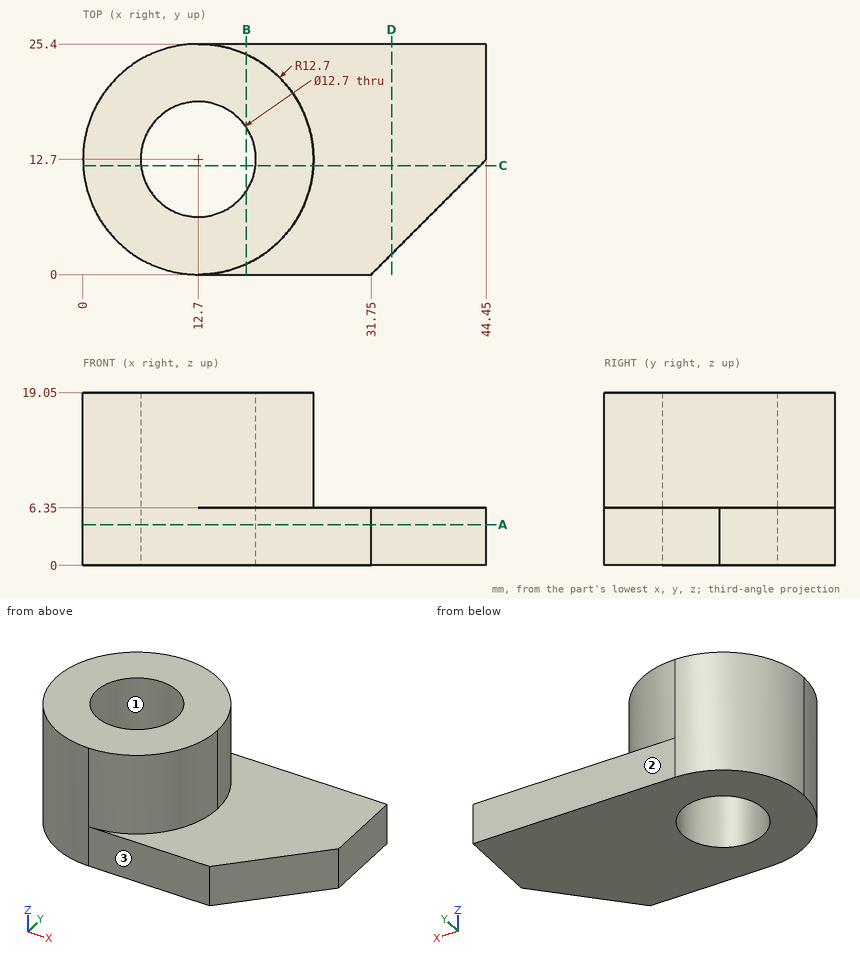
Geometry: see drawing. Coordinates: mm, zero at the bounding-box minimum. Coordinates: 2 decimals unless noted, no trailing zeros. Order: outer loops, then holes, each group sorted by start corner. A loop starts at its lowest first (then second) coordinate and runs counter-clockwise, first axis right, second up. Notation, with made-up numbers: M 85.25,17 L 89.25,17 A15 ccw 89.25,40 Z; hole C 88,81.5 d9. An arc over 180 degrees is marked long. Write each question's results on one line, items separated by ' | '. Start each with the question number.
1) Section query A-A (z = 4.5). Return the cut outline in (x, y).
2) Line query: line 1 (Z direction, x = 25, y = 7.25); line 2 (X direction, y = 13.5, z = 7); line 3 (Y direction, x = 18, z = 5.25). Output: solid intervals per line, ascending. Write a range as from..to.
3) Section query B-B (x = 18). Return the cut outline in (y, z).
4) Section query D-D (x = 34). Return the cut outline in (y, z), plus the area to 3 significant figures.
5) Draft query along Y for the marked faces 1, 2 and 3. Return one class per face: released by +Y, released by -Y, zero draft, split by the parting line, or undercut.
6) Contact query for flat-ended pins moving along their axis: pin 1 Ø3 at (y, z) = (16.5, 3.5) entering from -X; pin 2 Ø4 at (y, z) = (13.5, 13) entering from +X; pin 3 Ø1 at (x, z) = (23, 8) entering from +Y; pin 4 Ø1 at (x, y) = (17, 16.5) entering from +Z. Output: stop coordinate, or through.
7) Section query C-C (y = 12). Return the cut outline in (x, z).
Answers:
1) outline: M 12.7,0 L 31.75,0 L 44.45,12.7 L 44.45,25.4 L 12.7,25.4 A12.7 ccw Z; hole C 12.7,12.7 d12.7
2) line 1: z = 0..6.35 | line 2: x = 0.03..6.4, 19..25.37 | line 3: y = 0..9.2, 16.2..25.4
3) outline: M 0,0 L 9.2,0 L 9.2,19.05 L 1.16,19.05 L 1.16,6.35 L 0,6.35 Z; M 16.2,0 L 25.4,0 L 25.4,6.35 L 24.24,6.35 L 24.24,19.05 L 16.2,19.05 Z
4) outline: M 2.25,0 L 25.4,0 L 25.4,6.35 L 2.25,6.35 Z | area: 147 mm^2
5) face 1: undercut | face 2: released by +Y | face 3: released by -Y
6) pin 1: stops at x = 0.21 | pin 2: stops at x = 25.4 | pin 3: stops at y = 20.78 | pin 4: passes through
7) outline: M 0.02,0 L 6.39,0 L 6.39,19.05 L 0.02,19.05 Z; M 19.01,0 L 43.75,0 L 43.75,6.35 L 25.38,6.35 L 25.38,19.05 L 19.01,19.05 Z
